Source: CAD feature listing. Evaluate the final solid. Frame: model axes, mm. Round coordinates to 2 decimals unless told otherwise and drop trailing zeros. Order: outer loops, then holes, each group sorted by start corner. A loop starts at its lowest first (then second) coordinate and runs counter-clockwise, first axis right, second up. Notation, with made-up numbers: (-14.5, 82.25) - (3.5, 82.25) arc R7 cw to (3.5, 92.25) - close; hole circle Ø6 at (54, -12). An arc over 180 degrees is marked (long way). Put each result on its own line as item: value. Start each with the question number.
1) Section B-B on x = 70.9. Output: boundary loops of the cut face in (y, z).
2) Line query: probe 1 along Z at (x, y) = (70.9, -21); probe 2 along X at (y, z) = (-28.5, 20.75); probe 3 along Z at (x, y) = (72.25, -28). Output: solid intervals per line, ascending. Write a range as [from, to].
3) Section C-C on z = 21.25. Output: boundary loops of the cut face in (x, y), then the cut area to 3 significant figures.
4) Contact query for flat-ended pins moving along their axis: P1, Ø4, axis at y = -5.5, z = 15.5, coming from the +X side; P2, Ø1, axis at x = 65.5, y = -8, coming from the -Z side; P3, Ø1.5, axis at x = 72, z = 17.5, coming from the +Y side; P4, Ø1.5, axis at y = -12.5, z = 21, coming from the +X side. Output: stop coordinate, or through.
5) Section A-A on y = -14.5. Output: boundary loops of the cut face in (x, z) (3 decimals), then the cut area to 3 significant figures.
6) Section D-D on x = 76.25. Output: boundary loops of the cut face in (y, z).
7) Mould query, pull axis Z, two halves, no side actions, for faces 1 (the face through (73, -12, 12.75)), 2 (the face through (64.22, -12.07, 19.93)), 3 (the face through (66.8, -12.1, 21.4)). Classes: +Z half, -Z half, draft (parallel to the pull), parting line (faces both ways), or undercut.
```python
from build123d import *

# Parameters (mm, degrees)
ESBO_O1_R                = 2.79
RESSALTO_EXTRUS_O1_DEPTH = 45.5


with BuildPart() as part:
    # Esboço1 → Ressalto-extrusão1 (new body)
    with BuildSketch(Plane.XZ.offset(34.5)):
        with BuildLine():
            Line((77.062658774, 17.174038106), (78.116878365, 19))
            Line((78.116878365, 19), (77.062658774, 20.825961894))
            ThreePointArc((77.062658774, 20.825961894), (75.013620668, 21.375), (75.562658774, 23.424038106))
            Line((75.562658774, 23.424038106), (74.508439182, 25.25))
            Line((74.508439182, 25.25), (72.4, 25.25))
            ThreePointArc((72.4, 25.25), (70.9, 23.75), (69.4, 25.25))
            Line((69.4, 25.25), (67.291560818, 25.25))
            Line((67.291560818, 25.25), (66.237341226, 23.424038106))
            ThreePointArc((66.237341226, 23.424038106), (66.786379332, 21.375), (64.737341226, 20.825961894))
            Line((64.737341226, 20.825961894), (63.683121635, 19))
            Line((63.683121635, 19), (64.737341226, 17.174038106))
            ThreePointArc((64.737341226, 17.174038106), (66.786379332, 16.625), (66.237341226, 14.575961894))
            Line((66.237341226, 14.575961894), (67.291560818, 12.75))
            Line((67.291560818, 12.75), (69.4, 12.75))
            ThreePointArc((69.4, 12.75), (70.9, 14.25), (72.4, 12.75))
            Line((72.4, 12.75), (74.508439182, 12.75))
            Line((74.508439182, 12.75), (75.562658774, 14.575961894))
            ThreePointArc((75.562658774, 14.575961894), (75.013620668, 16.625), (77.062658774, 17.174038106))
        make_face()
        with Locations((70.9, 19)):
            Circle(ESBO_O1_R, mode=Mode.SUBTRACT)
    extrude(amount=-RESSALTO_EXTRUS_O1_DEPTH)


solid = part.part
```
Answer sheet:
1. outline: (-34.5, 14.25) - (11, 14.25) - (11, 16.21) - (-34.5, 16.21) - close; (-34.5, 21.79) - (11, 21.79) - (11, 23.75) - (-34.5, 23.75) - close
2. probe 1: [14.25, 16.21], [21.79, 23.75]
2. probe 2: [64.69, 64.89], [66.09, 68.73], [73.07, 75.71], [76.91, 77.11]
2. probe 3: [13.4, 16.56], [21.44, 24.6]
3. outline: (66.71, -34.5) - (69.25, -34.5) - (69.25, 11) - (66.71, 11) - close; (72.55, -34.5) - (75.09, -34.5) - (75.09, 11) - (72.55, 11) - close
3. area: 232 mm^2
4. P1: x = 77.25
4. P2: z = 17.28
4. P3: through
4. P4: x = 77.4
5. outline: (63.683, 19) - (64.737, 17.174) arc R1.5 cw to (66.237, 14.576) - (67.292, 12.75) - (69.4, 12.75) arc R1.5 cw to (72.4, 12.75) - (74.508, 12.75) - (75.563, 14.576) arc R1.5 cw to (77.063, 17.174) - (78.117, 19) - (77.063, 20.826) arc R1.5 cw to (75.563, 23.424) - (74.508, 25.25) - (72.4, 25.25) arc R1.5 cw to (69.4, 25.25) - (67.292, 25.25) - (66.237, 23.424) arc R1.5 cw to (64.737, 20.826) - close; hole circle Ø5.58 at (70.9, 19)
5. area: 89.7 mm^2
6. outline: (-34.5, 17.37) - (11, 17.37) - (11, 20.63) - (-34.5, 20.63) - close
7. face 1: -Z half
7. face 2: +Z half
7. face 3: undercut
